For this review, take the finished solid that the model builds, in its own axes (mm). Give positions to 0.01 mm unless a question says otherwise; leave off trailing zeros. Loops run counter-clockwise (first coordinate to the right, second up) from the corner with the lowest first, then second, coordinate; pieces in that order, holes last. Notation, with made-up numbers: (9.25, 10.25) - (40.25, 10.25) arc R17 cw to (40.25, 28.25) - close; hole circle Ø3 at (0, 33.25). An arc over 180 degrees is marked (long way). Put each result on its own line as item: value.
from build123d import *

# Parameters (mm, degrees)
SKETCH_1_R      = 1.5
EXTRUDE_1_DEPTH = 3


with BuildPart() as part:
    # 草图1 → 凸台-拉伸1 (new body)
    with BuildSketch(Plane(origin=(0, 0, 0), x_dir=(1, 0, 0), z_dir=(0, 1, 0))):
        Polygon((0, 0), (0, 5.286885246), (-20, 5.286885246), (-20, -4.713114754), (0, -4.713114754), align=None)
        with Locations((-18, 0.286885246)):
            Circle(SKETCH_1_R, mode=Mode.SUBTRACT)
        with Locations((-2, 0.286885246)):
            Circle(SKETCH_1_R, mode=Mode.SUBTRACT)
    extrude(amount=EXTRUDE_1_DEPTH)


solid = part.part
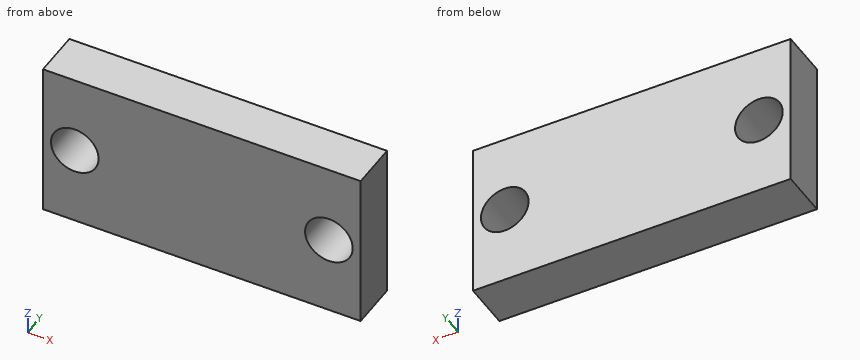
1) Take a section at B-B on x = -1.5. State the section outline as (y, z) points.
Geometry check:
outline: (0, -5.29) - (3, -5.29) - (3, -1.7) - (0, -1.7) - close; (0, 1.13) - (3, 1.13) - (3, 4.71) - (0, 4.71) - close
2) Take a section at A-A on x = -18. State the section outline as (y, z) points, and give its area (3 significant figures).
Geometry check:
outline: (0, -5.29) - (3, -5.29) - (3, -1.79) - (0, -1.79) - close; (0, 1.21) - (3, 1.21) - (3, 4.71) - (0, 4.71) - close
area: 21.0 mm²
3) Insertion check: pin 1 Ø1.8 at (x, z) = (-18, -0.29) entering from -Y. The pin has a flat end and moves straight along its axis. Give the tip position at first contact, or say it passes through.
Geometry check:
pin 1: passes through
4) Wall thickness on line 1 (Z direction, x = -2, y = 1.7); line 2 (X direction, y = 0.8, z = 1); line 3 (X direction, y = 1.9, z = 0.25): over which ranges is each line inside the solid? List them lowest first.
Geometry check:
line 1: z = -5.29 to -1.79, 1.21 to 4.71
line 2: x = -20 to -18.77, -17.23 to -2.77, -1.23 to 0
line 3: x = -20 to -19.4, -16.6 to -3.4, -0.6 to 0
5) Take a section at C-C on y = 1.15. State the section outline as (x, z) points, and give its area (3 significant figures).
Geometry check:
outline: (-20, -5.29) - (0, -5.29) - (0, 4.71) - (-20, 4.71) - close; hole circle Ø3 at (-18, -0.29); hole circle Ø3 at (-2, -0.29)
area: 186 mm²
